Read the model definition and answer for the solid it produces. Units are mm, in the model's axes. Face numbers are marked on the shaded views. Coordinates: 2 decimals unless noted, no trailing zeros. Order: outer loops, then holes, each group sorted by start corner. A loop starts at its lowest first (then second) coordinate and runs counter-clockwise, first axis right, second up.
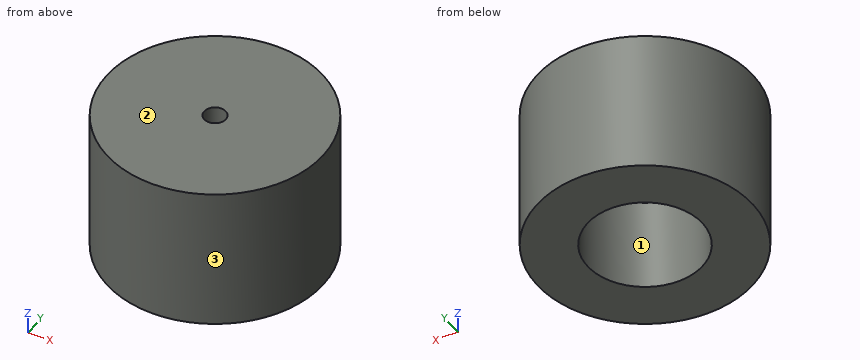
from build123d import *

# Parameters (mm, degrees)
CROQUIS1_R              = 15
SALIENTE_EXTRUIR1_DEPTH = 20
CROQUIS2_R              = 8
CORTAR_EXTRUIR1_DEPTH   = 13
CORTAR_EXTRUIR2_REACH   = 31.155
CROQUIS3_R              = 1.5


with BuildPart() as part:
    # Croquis1 → Saliente-Extruir1 (new body)
    with BuildSketch(Plane.XY):
        Circle(CROQUIS1_R)
    extrude(amount=SALIENTE_EXTRUIR1_DEPTH)

    # Croquis2 → Cortar-Extruir1 (cut)
    with BuildSketch(Plane(origin=(0, 0, 0), x_dir=(-1, 0, 0), z_dir=(0, 0, -1))):
        Circle(CROQUIS2_R)
    extrude(amount=-CORTAR_EXTRUIR1_DEPTH, mode=Mode.SUBTRACT)

    # Croquis3 → Cortar-Extruir2 (cut, up to next)
    with BuildSketch(Plane.XY.offset(20), mode=Mode.PRIVATE) as cortar_extruir2_sk1:
        Circle(CROQUIS3_R)
    cortar_extruir2_tool1 = extrude(cortar_extruir2_sk1.sketch, amount=-CORTAR_EXTRUIR2_REACH, mode=Mode.PRIVATE) & part.part
    add(cortar_extruir2_tool1.solids().sort_by_distance((0, 0, 20))[0], mode=Mode.SUBTRACT)


solid = part.part
Q1. Each of these flat-tipped pins is pushed along its axis until it touches: P1, Ø6, axis at y = 11, z = 15.5, coming from the -X side; P2, Ø5, axis at x = -3.5, z = 5.5, coming from the +Y side; P3, Ø8, axis at y = -9.5, z = 16.5, coming from the +X side; P4, Ø10, axis at y = -4.5, z = 10, coming from the -X side. Where does it stop, or does it pass through?
Q2. The part is cut by section C-C, the plane z = 1.5. Determine the outline of the cut face in (x, y), then the cut area to 3 significant figures.
Q3. The part is cut by section A-A, the plane x = 0. Determine the outline of the cut face in (y, z).
Q4. Determine the mould class of the marked faces 1, 2 and 3 for opening direction Y: +Y half, -Y half, draft (parallel to the pull), parting line (faces both ways), or undercut.
Q5. Straight lines are drawn through the part: L1, parallel to Y at x = 0, z = 5.5; L2, parallel to Y at x = 1, z = 9.5; L3, parallel to Z at x = 3.25, y = -4.5. For each, find the intervals that lie inside material, in ascending order.
Q6. The part is cut by section D-D, the plane x = 7.25. Determine the outline of the cut face in (y, z).
Computed values:
1. P1: stops at x = -12.69
1. P2: stops at y = 14.97
1. P3: stops at x = 13.96
1. P4: stops at x = -15
2. outline: circle Ø30 at (0, 0); hole circle Ø16 at (0, 0)
2. area: 506 mm2
3. outline: (-15, 0) - (-8, 0) - (-8, 13) - (-1.5, 13) - (-1.5, 20) - (-15, 20) - close; (1.5, 13) - (8, 13) - (8, 0) - (15, 0) - (15, 20) - (1.5, 20) - close
4. face 1: undercut
4. face 2: draft
4. face 3: parting line
5. L1: y = -15 to -8, 8 to 15
5. L2: y = -14.97 to -7.94, 7.94 to 14.97
5. L3: z = 13 to 20
6. outline: (-13.13, 0) - (-3.38, 0) - (-3.38, 13) - (3.38, 13) - (3.38, 0) - (13.13, 0) - (13.13, 20) - (-13.13, 20) - close
